from build123d import *

# Parameters (mm, degrees)
F0_W           = 25
F0_H           = 12
F0_W_2         = 19
F0_H_2         = 8
F1_DEPTH       = 10
F2_W           = 21
F2_H           = 8
F2_W_2         = 17
F2_H_2         = 2
F3_DEPTH       = 25
F4_W           = 21
F4_H           = 8
F4_W_2         = 17
F4_H_2         = 2
F5_DEPTH       = 2
F6_W           = 25
F6_H           = 12
F7_DEPTH       = 4
F10_DEPTH      = 4
F10_DEPTH_BACK = 4
F11_T1_DEPTH   = 21
F11_T3_DEPTH   = 8
F11_T9_DEPTH   = 31
F11_T14_DEPTH  = 18
F11_T22_DEPTH  = 31
F11_T27_DEPTH  = 18
F11_T35_DEPTH  = 31
F11_T40_DEPTH  = 18
F11_T48_DEPTH  = 18
F11_T53_DEPTH  = 31
F12_R          = 1
F14_DEPTH      = 1


# Not quite as in the source:
# - a fillet or chamfer that OpenCascade refuses, or shapes differently, is made with other operations: its cross-section is extruded or revolved along the edge and cut away or added


with BuildPart() as f1:
    # F0 (on Top) → F1 (new body)
    with BuildSketch(Plane.XY):
        with Locations((12.5, 6)):
            Rectangle(F0_W, F0_H)
        with Locations((12.5, 6)):
            Rectangle(F0_W_2, F0_H_2, mode=Mode.SUBTRACT)
    extrude(amount=-F1_DEPTH)

    # F2 (on Top) → F3 (join)
    with BuildSketch(Plane.XY):
        with Locations((12.5, 6)):
            Rectangle(F2_W, F2_H)
        with Locations((12.5, 6)):
            Rectangle(F2_W_2, F2_H_2, mode=Mode.SUBTRACT)
    extrude(amount=F3_DEPTH)

    # F4 (on face) → F5 (join)
    with BuildSketch(Plane.XY.offset(25)):
        with Locations((12.5, 6)):
            Rectangle(F4_W, F4_H)
        with Locations((12.5, 6)):
            Rectangle(F4_W_2, F4_H_2, mode=Mode.SUBTRACT)
        with Locations((12.5, 6)):
            Rectangle(F4_W_2, F4_H_2)
    extrude(amount=F5_DEPTH)

    # F6 (on face) → F7 (join)
    with BuildSketch(Plane.XY):
        with Locations((12.5, 6)):
            Rectangle(F6_W, F6_H)
        Polygon((23, 2), (22, 2), (3, 2), (2, 2), (2, 10), (3, 10), (22, 10), (23, 10), align=None, mode=Mode.SUBTRACT)
    extrude(amount=F7_DEPTH)

    # F9 (on offset) → F10 (join, two sides)
    with BuildSketch(Plane.XZ.offset(-6)) as f10_sk:
        with BuildLine():
            Line((3, -7), (3, -8.5))
            Line((3, -8.5), (3.4671572875, -8.0328427125))
            ThreePointArc((3.4671572875, -8.0328427125), (3.5843145751, -7.75), (3.4671572875, -7.4671572875))
            Line((3.4671572875, -7.4671572875), (3, -7))
        make_face()
        with BuildLine():
            Line((21.5328427125, -8.0328427125), (22, -8.5))
            Line((22, -8.5), (22, -7))
            Line((22, -7), (21.5328427125, -7.4671572875))
            ThreePointArc((21.5328427125, -7.4671572875), (21.4156854249, -7.75), (21.5328427125, -8.0328427125))
        make_face()
    extrude(amount=F10_DEPTH)
    extrude(f10_sk.sketch, amount=-F10_DEPTH_BACK)

    # F11: fillet of radius 5 on 4 edges, made by hand

    # F11_s2 → F11_t1 (join)
    with BuildSketch(Plane.YZ.offset(2)):
        with BuildLine():
            ThreePointArc((0, 4), (1.472135955, 5.7639320225), (2, 8))
            Line((2, 8), (2, 4))
            Line((2, 4), (0, 4))
        make_face()
        with BuildLine():
            ThreePointArc((12, 4), (10.527864045, 5.7639320225), (10, 8))
            Line((10, 8), (10, 4))
            Line((10, 4), (12, 4))
        make_face()
    extrude(amount=F11_T1_DEPTH)

    # F11_s4 → F11_t3 (join)
    with BuildSketch(Plane.XZ.offset(-10)):
        with BuildLine():
            ThreePointArc((25, 4), (23.527864045, 5.7639320225), (23, 8))
            Line((23, 8), (23, 4))
            Line((23, 4), (25, 4))
        make_face()
        with BuildLine():
            ThreePointArc((0, 4), (1.472135955, 5.7639320225), (2, 8))
            Line((2, 8), (2, 4))
            Line((2, 4), (0, 4))
        make_face()
    extrude(amount=F11_T3_DEPTH)


with BuildPart() as f11_tool7:
    # F11_s8 → F11_t9 (new body)
    with BuildSketch(Plane.YZ.offset(-8)):
        with BuildLine():
            ThreePointArc((0, 4), (1.472135955, 5.7639320225), (2, 8))
            Line((2, 8), (2, 4))
            Line((2, 4), (0, 4))
        make_face()
    extrude(amount=F11_T9_DEPTH)

    split(bisect_by=Plane.YZ, keep=Keep.TOP)

    split(bisect_by=Plane.YZ.offset(2), keep=Keep.BOTTOM)


with BuildPart() as f11_tool12:
    # F11_s13 → F11_t14 (new body)
    with BuildSketch(Plane.XZ.offset(8)):
        with BuildLine():
            ThreePointArc((0, 4), (1.472135955, 5.7639320225), (2, 8))
            Line((2, 8), (2, 4))
            Line((2, 4), (0, 4))
        make_face()
    extrude(amount=-F11_T14_DEPTH)

    split(bisect_by=Plane.XZ, keep=Keep.BOTTOM)

    split(bisect_by=Plane.XZ.offset(-2), keep=Keep.TOP)


with BuildPart() as f11_tool7_1:
    add(f11_tool7.part)

    # F11_t17: intersect F11_tool12
    add(f11_tool12.part, mode=Mode.INTERSECT)


with BuildPart() as f1_1:
    add(f1.part)

    # F11_t5: union F11_tool7
    add(f11_tool7_1.part)


with BuildPart() as f11_tool20:
    # F11_s21 → F11_t22 (new body)
    with BuildSketch(Plane.YZ.offset(2)):
        with BuildLine():
            ThreePointArc((0, 4), (1.472135955, 5.7639320225), (2, 8))
            Line((2, 8), (2, 4))
            Line((2, 4), (0, 4))
        make_face()
    extrude(amount=F11_T22_DEPTH)

    split(bisect_by=Plane.YZ.offset(25), keep=Keep.BOTTOM)

    split(bisect_by=Plane.YZ.offset(23), keep=Keep.TOP)


with BuildPart() as f11_tool25:
    # F11_s26 → F11_t27 (new body)
    with BuildSketch(Plane.XZ.offset(-10)):
        with BuildLine():
            ThreePointArc((25, 4), (23.527864045, 5.7639320225), (23, 8))
            Line((23, 8), (23, 4))
            Line((23, 4), (25, 4))
        make_face()
    extrude(amount=F11_T27_DEPTH)

    split(bisect_by=Plane.XZ, keep=Keep.BOTTOM)

    split(bisect_by=Plane.XZ.offset(-2), keep=Keep.TOP)


with BuildPart() as f11_tool20_1:
    add(f11_tool20.part)

    # F11_t30: intersect F11_tool25
    add(f11_tool25.part, mode=Mode.INTERSECT)


with BuildPart() as f1_2:
    add(f1_1.part)

    # F11_t18: union F11_tool20
    add(f11_tool20_1.part)


with BuildPart() as f11_tool33:
    # F11_s34 → F11_t35 (new body)
    with BuildSketch(Plane.YZ.offset(33)):
        with BuildLine():
            ThreePointArc((12, 4), (10.527864045, 5.7639320225), (10, 8))
            Line((10, 8), (10, 4))
            Line((10, 4), (12, 4))
        make_face()
    extrude(amount=-F11_T35_DEPTH)

    split(bisect_by=Plane.YZ.offset(25), keep=Keep.BOTTOM)

    split(bisect_by=Plane.YZ.offset(23), keep=Keep.TOP)


with BuildPart() as f11_tool38:
    # F11_s39 → F11_t40 (new body)
    with BuildSketch(Plane.XZ.offset(-20)):
        with BuildLine():
            ThreePointArc((25, 4), (23.527864045, 5.7639320225), (23, 8))
            Line((23, 8), (23, 4))
            Line((23, 4), (25, 4))
        make_face()
    extrude(amount=F11_T40_DEPTH)

    split(bisect_by=Plane.XZ.offset(-12), keep=Keep.TOP)

    split(bisect_by=Plane.XZ.offset(-10), keep=Keep.BOTTOM)


with BuildPart() as f11_tool33_1:
    add(f11_tool33.part)

    # F11_t43: intersect F11_tool38
    add(f11_tool38.part, mode=Mode.INTERSECT)


with BuildPart() as f1_3:
    add(f1_2.part)

    # F11_t31: union F11_tool33
    add(f11_tool33_1.part)


with BuildPart() as f11_tool46:
    # F11_s47 → F11_t48 (new body)
    with BuildSketch(Plane.XZ.offset(-2)):
        with BuildLine():
            ThreePointArc((0, 4), (1.472135955, 5.7639320225), (2, 8))
            Line((2, 8), (2, 4))
            Line((2, 4), (0, 4))
        make_face()
    extrude(amount=-F11_T48_DEPTH)

    split(bisect_by=Plane.XZ.offset(-12), keep=Keep.TOP)

    split(bisect_by=Plane.XZ.offset(-10), keep=Keep.BOTTOM)


with BuildPart() as f11_tool51:
    # F11_s52 → F11_t53 (new body)
    with BuildSketch(Plane.YZ.offset(23)):
        with BuildLine():
            ThreePointArc((12, 4), (10.527864045, 5.7639320225), (10, 8))
            Line((10, 8), (10, 4))
            Line((10, 4), (12, 4))
        make_face()
    extrude(amount=-F11_T53_DEPTH)

    split(bisect_by=Plane.YZ, keep=Keep.TOP)

    split(bisect_by=Plane.YZ.offset(2), keep=Keep.BOTTOM)


with BuildPart() as f11_tool46_1:
    add(f11_tool46.part)

    # F11_t56: intersect F11_tool51
    add(f11_tool51.part, mode=Mode.INTERSECT)


with BuildPart() as f1_4:
    add(f1_3.part)

    # F11_t44: union F11_tool46
    add(f11_tool46_1.part)

    # F12
    f12_edges = [f1_4.edges().sort_by_distance(p)[0] for p in [
        (23, 6, 27),
        (12.5, 2, 27),
        (2, 6, 27),
        (12.5, 10, 27),
        (12.5, 12, 4),
        (25, 6, 4),
        (12.5, 0, 4),
        (0, 6, 4),
    ]]
    fillet(f12_edges, radius=F12_R)

    # F13 (on face) → F14 (cut)
    with BuildSketch(Plane(origin=(0, 10, 0), x_dir=(-1, 0, 0), z_dir=(0, 1, 0))):
        Polygon((-12.5, 20.9), (-17, 13.1057713659), (-8, 13.1057713659), align=None)
        Polygon((-16.1339745962, 13.6057713659), (-14.4613248654, 16.502885683), (-12.7886751346, 13.6057713659), align=None, mode=Mode.SUBTRACT)
        Polygon((-12.5, 13.6057713659), (-14.3169872981, 16.752885683), (-10.6830127019, 16.752885683), align=None, mode=Mode.SUBTRACT)
        Polygon((-8.8660254038, 13.6057713659), (-12.2113248654, 13.6057713659), (-10.5386751346, 16.502885683), align=None, mode=Mode.SUBTRACT)
        Polygon((-12.5, 19.9), (-10.8273502692, 17.002885683), (-14.1726497308, 17.002885683), align=None, mode=Mode.SUBTRACT)
    extrude(amount=-F14_DEPTH, mode=Mode.SUBTRACT)


solid = f1_4.part
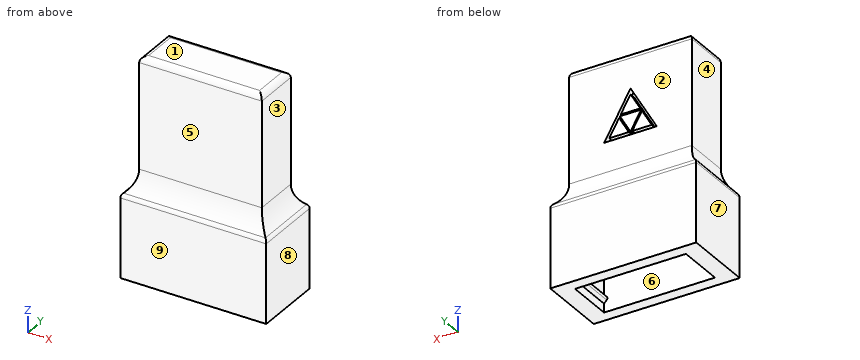
Geometry check sheet. Reference: the model listing, model coordinates, mm. Face numbers are marked on the shaded views. A direction names the side the tool comes from. Round coordinates to 2 decimals unless told otherwise and drop trailing zeros. Loops run counter-clockwise (first coordinate to the right, second up) from the corner with the lowest first, then second, coordinate; pieces in that order, holes last.
Item 1: Cross-section at C-C on x = 17.75. Record the boundary of the cut face in (y, z), then the cut area to 3 significant figures.
Item 2: Thickness scan on line 1 (X direction, y = 7.75, z = -3); line 2 (Y direction, x = 20.75, z = -2); line 3 (X direction, y = 6, z = 10.5). Record the ranges inside material, lowest first.
Item 3: Gauge pin test, flat ends, axial feed: pin 1 (1.6 mm diameter, centred on y = 6.5, z = 7, fed in from +X); pin 2 (6.5 mm diameter, centred on y = 4.5, z = 12.5, fed in from +X); pin 3 (4 mm diameter, centred on x = 13, z = 17.5, fed in from +Y). Record the tip position at first contact, or that the pin passes through.
Item 4: Cross-section at A-A on z = 22. Record the boundary of the cut face in (x, y).
Item 5: Cross-section at B-B on y = 6.25. Record the boundary of the cut face in (x, z).
Item 6: Cross-section at D-D on y = 3.5. Record the boundary of the cut face in (x, z), then the cut area to 3 significant figures.
Item 7: Access from +Z, -Z, +X, -X, +Y, -Y to the whole of each face (thin tool, end or side, straight path). Record for the marked faces 1, 2, 3, 4 and 5.
Item 8: Mould release check, pull along X, two halves, no side actions. Record for the marked faces 6, 7, 8 and 9: pulls with the +X half, pulls with the -X half, needs draft (parallel to the pull), parting line crosses it, or undercut.
Answer sheet:
1. outline: (0, -10) - (2, -10) - (2, 0) - (5, 0) - (5, 25) - (7, 25) - (7, 0) - (10, 0) - (10, -10) - (12, -10) - (12, 3.53) arc R1 ccw to (11.67, 4.27) arc R5 cw to (10, 8) - (10, 26) arc R1 ccw to (9, 27) - (3, 27) arc R1 ccw to (2, 26) - (2, 8) arc R5 cw to (0.33, 4.27) arc R1 ccw to (0, 3.53) - close
1. area: 226 mm2
2. line 1: x = 0 to 3, 22 to 25
2. line 2: y = 0 to 2, 10 to 12
2. line 3: x = 2 to 4, 21 to 23
3. pin 1: stops at x = 23.34
3. pin 2: stops at x = 23
3. pin 3: stops at y = 10
4. outline: (2, 2) - (23, 2) - (23, 10) - (2, 10) - close; hole (4, 5) - (21, 5) - (21, 7) - (4, 7) - close
5. outline: (0, -10) - (3, -10) - (3, -8.5) - (3.47, -8.03) arc R0.4 ccw to (3.47, -7.47) - (3, -7) - (3, 0) - (4, 0) - (4, 25) - (21, 25) - (21, 0) - (22, 0) - (22, -7) - (21.53, -7.47) arc R0.4 ccw to (21.53, -8.03) - (22, -8.5) - (22, -10) - (25, -10) - (25, 3.53) arc R1 ccw to (24.67, 4.27) arc R5 cw to (23, 8) - (23, 26) arc R1 ccw to (22, 27) - (3, 27) arc R1 ccw to (2, 26) - (2, 8) arc R5 cw to (0.33, 4.27) arc R1 ccw to (0, 3.53) - close
6. outline: (0, -10) - (3, -10) - (3, -8.5) - (3.47, -8.03) arc R0.4 ccw to (3.47, -7.47) - (3, -7) - (3, 0) - (22, 0) - (22, -7) - (21.53, -7.47) arc R0.4 ccw to (21.53, -8.03) - (22, -8.5) - (22, -10) - (25, -10) - (25, 3.53) arc R1 ccw to (24.67, 4.27) arc R5 cw to (23, 8) - (23, 26) arc R1 ccw to (22, 27) - (3, 27) arc R1 ccw to (2, 26) - (2, 8) arc R5 cw to (0.33, 4.27) arc R1 ccw to (0, 3.53) - close
6. area: 648 mm2
7. face 1: +Z, +X, -X, +Y, -Y
7. face 2: +Z, +X, -X, +Y
7. face 3: +Z, +X, +Y, -Y
7. face 4: +Z, -X, +Y, -Y
7. face 5: +Z, +X, -X, -Y
8. face 6: undercut
8. face 7: pulls with the -X half
8. face 8: pulls with the +X half
8. face 9: needs draft
